Autodesk Inventor part; units mm, degrees
ref_plane "YZ Plane" through (0, 0, 0) normal (1, 0, 0) x (0, 1, 0)
ref_plane "XZ Plane" through (0, 0, 0) normal (0, 1, 0) x (-1, 0, 0)
ref_plane "XY Plane" through (0, 0, 0) normal (0, 0, 1) x (1, 0, 0)
sketch "Sketch1" plane through (0, 0, 0) normal (0, 0, 1) x (1, 0, 0)
  circle A0 centre (0, 0) radius 4.25
  circle A1 centre (0, 0) radius 3.5
  circle A2 centre (0, 0) radius 5.5
  circle A3 centre (0, 0) radius 3.4
  dimension "d0" = 8.5
  dimension "d1" = 7
  dimension "d2" = 11
  dimension "d23" = 6.8
extrude "Extrusion1" add sketch "Sketch1" along normal blind 2.5 contours A2
extrude "Extrusion6" add sketch "Sketch1" along normal blind 6 contours A0 | A1
fillet "Fillet4" radius 0.4 2 edges at (-3.4, 0, 6) (-4.25, 0, 6)
extrude "Extrusion13" cut sketch "Sketch1" along normal blind 1.5 contours A1
properties part number "SmaRing_2.5mm_3.5mm_6.8mm"
CAD build for the part. Positions are in the model's coordinates, mm. A direction names the side the tool comes from. Coordinates: 2 decimals unless noted, no trailing zeros. Write each loop counter-clockwise with the first axis right and the second up, starting at its lowest first coordinate (ties: lowest second). Pieces come first, ordered by that corner, then holes. Notation, with made-up numbers: (73.5, 29) - (127.5, 29) arc R15 cw to (127.5, 51) - close; hole circle Ø1 at (55.25, -14). An arc over 180 degrees is marked (long way). Use a Markdown table: item, result. Add a question column.
Item 1: Band-saw the part on A-A, the plane y = 0. Give the cut face in (x, z), and give its area (3 significant figures).
Item 2: Mould opens along X. For faces 3 (the face through (-0.74, 3.32, 3.52)), 4 (the face through (-1.19, 5.37, 1.23)), 5 (the face through (4, 0, 0)) say: pulls with the +X half, pulls with the -X half, needs draft (parallel to the pull), parting line crosses it, or undercut.
Item 3: Drill centre lines: L1, parallel to Y at x = 0, z = 0.9; L2, parallel to Y at x = 0, z = 4.65; L3, parallel to Z at x = -0.5, y = 4.75. Where is each one in solid material? Low to high. Write a range as from..to.
Item 4: Flat gauge pins, fed straight in: pin 1 (6.5 mm diameter, centred on x = 0, y = 0, fed in from -Z); pin 2 (1 mm diameter, centred on x = -4, z = 1.5, fed in from +Y). Where does each tip first touch, or does it go through?
Item 5: Band-saw the part on D-D, the plane y = 4.5. Give the cut face in (x, z), and give its area (3 significant figures).
Item 6: 3-axis set-ups, long thin cutter, end or side, ignore diameter. For faces 1 (the face through (3.233, 1.341, 0.74)), 2 (the face through (2, -4, 2.5)): which of +Z, -Z, +X, -X, +Y, -Y reach the whole face in a straight line?
Item 7: Band-saw the part on C-C, the plane z = 4.1. Give the cut face in (x, y).
Numbers:
| question | item | result |
|---|---|---|
| 1 | outline | (-5.5, 0) - (-3.5, 0) - (-3.5, 1.5) - (-3.4, 1.5) - (-3.4, 5.6) arc R0.4 ccw to (-3.8, 6) - (-3.85, 6) arc R0.4 ccw to (-4.25, 5.6) - (-4.25, 2.5) - (-5.5, 2.5) - close; (3.4, 1.5) - (3.5, 1.5) - (3.5, 0) - (5.5, 0) - (5.5, 2.5) - (4.25, 2.5) - (4.25, 5.6) arc R0.4 ccw to (3.85, 6) - (3.8, 6) arc R0.4 ccw to (3.4, 5.6) - close |
| 1 | area | 16.0 mm2 |
| 2 | face 3 | undercut |
| 2 | face 4 | parting line crosses it |
| 2 | face 5 | needs draft |
| 3 | L1 | -5.5..-3.5, 3.5..5.5 |
| 3 | L2 | -4.25..-3.4, 3.4..4.25 |
| 3 | L3 | 0..2.5 |
| 4 | pin 1 | through |
| 4 | pin 2 | y = 4.24 |
| 5 | outline | (-3.16, 0) - (3.16, 0) - (3.16, 2.5) - (-3.16, 2.5) - close |
| 5 | area | 15.8 mm2 |
| 6 | face 1 | -Z |
| 6 | face 2 | +Z |
| 7 | outline | circle Ø8.5 at (0, 0); hole circle Ø6.8 at (0, 0) |
